Job drawing, mm, ordinate dimensions from the low corner. One solid piece. A direction names the side the tool comes from. Round coordinates to 2 decimals unless told otherwise and drop trailing zeros. Loops run counter-clockwise (first coordinate to the right, second up) from the corner with the lowest first, then second, coordinate; pieces in that order, holes last. Notation, with made-up numbers: M 2,-18 L 30,-18 A32 ccw 30,10 Z; hole C 31.25,-9.75 d10. An arc over 180 degrees is marked long. Put each result on its own line as item: value. Start each with the question number.
1) Slice it at D-D on y = 19. Give the cut face in (x, z), then the cut area to 3 significant figures.
2) Which spindle directions (+Z, -Z, +X, -X, +Y, -Y) get a long thin tool onto all of the face, cutting with end or side? Do the marked faces 4, 5 and 6. Say none if no direction does.
3) Pull direction Z, two halves, no side cores. Call the marked faces 1, 2 and 3: +Z half, -Z half, draft (parallel to the pull), parting line (faces both ways), or undercut.
4) Slice it at A-A on y = 4. Give the cut face in (x, z), then the cut area to 3 significant figures.
5) Slice it at C-C on x = 7.5. Give the cut face in (y, z).
6) Drop flat-ended pins along their axis: pin 1 Ø1.2 at (y, z) = (25.5, 35.8) entering from -X; pin 2 Ø0.9 at (x, z) = (3.5, 73.5) entering from -Y; pin 3 Ø6 at (x, z) = (1.5, 52.5) entering from -Y; pin 4 Ø3.5 at (x, z) = (3.5, 82) entering from +Y. Give the stop position or say it passes through.
7) Slice it at B-B on z = 3. Give the cut face in (x, y).
8) Probe line 1 along X through (y, z) = (3.75, 11.75); line 2 along Z through (x, y) = (4, 13.5); line 3 along Y through (x, z) = (8.5, 62.6). List the from-to ranges inside material, lowest first.
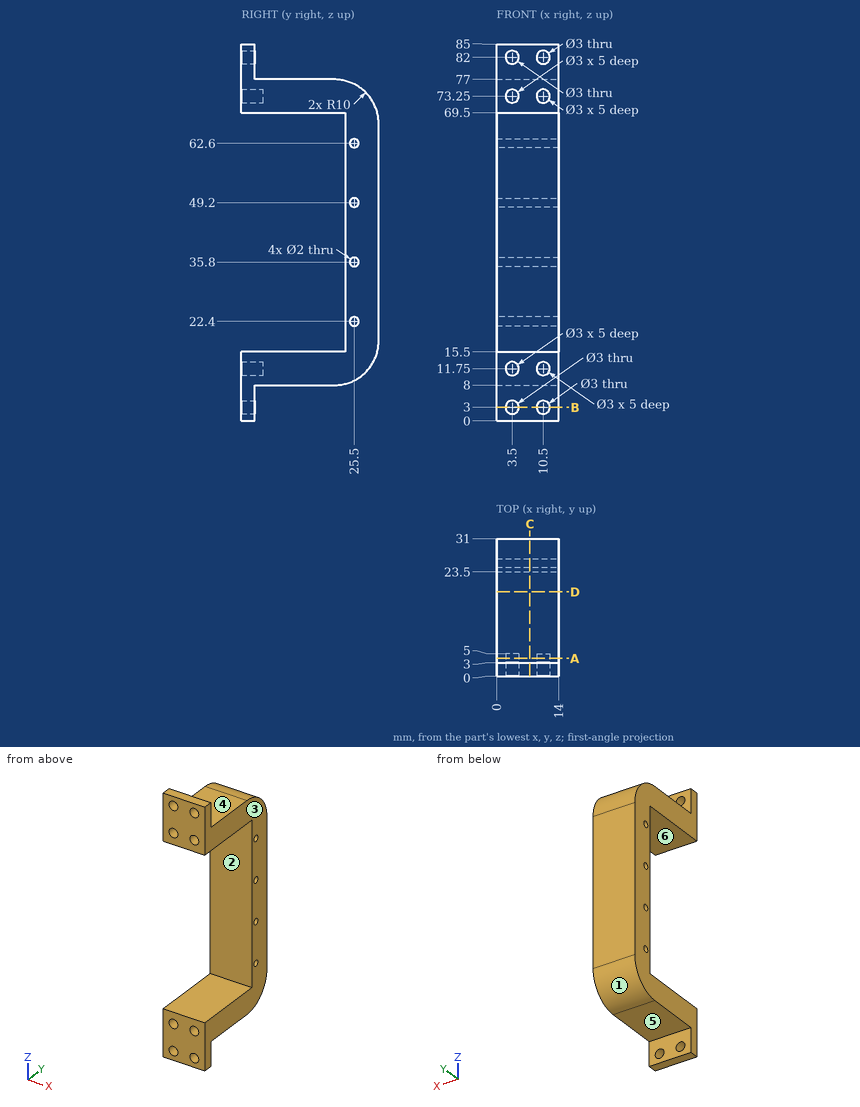
Recorded:
1. outline: M 0,8 L 14,8 L 14,15.5 L 0,15.5 Z; M 0,69.5 L 14,69.5 L 14,77 L 0,77 Z
1. area: 210 mm2
2. face 4: +Z, +X, -X, +Y
2. face 5: -Z, +X, -X, +Y
2. face 6: +X, -X, -Y
3. face 1: -Z half
3. face 2: undercut
3. face 3: draft
4. outline: M 0,8 L 14,8 L 14,15.5 L 0,15.5 Z; M 0,69.5 L 14,69.5 L 14,77 L 0,77 Z; hole C 3.5,11.75 d3; hole C 3.5,73.25 d3; hole C 10.5,11.75 d3; hole C 10.5,73.25 d3
4. area: 182 mm2
5. outline: M 0,0 L 3,0 L 3,8 L 21,8 A10 ccw 31,18 L 31,67 A10 ccw 21,77 L 3,77 L 3,85 L 0,85 L 0,69.5 L 23.5,69.5 L 23.5,15.5 L 0,15.5 Z; hole C 25.5,22.4 d2; hole C 25.5,35.8 d2; hole C 25.5,49.2 d2; hole C 25.5,62.6 d2
6. pin 1: passes through
6. pin 2: stops at y = 5
6. pin 3: stops at y = 23.5
6. pin 4: stops at y = 3
7. outline: M 0,0 L 2,0 L 2,3 L 0,3 Z; M 5,0 L 9,0 L 9,3 L 5,3 Z; M 12,0 L 14,0 L 14,3 L 12,3 Z
8. line 1: x = 0 to 2, 5 to 9, 12 to 14
8. line 2: z = 8 to 15.5, 69.5 to 77
8. line 3: y = 23.5 to 24.5, 26.5 to 31
